Could you check a few things on this model? Use its own coordinates, in mm. A direction names the side the tool comes from. Round coordinates to 2 decimals unless told otherwise and drop trailing zeros. Order: outer loops, then holes, each group sorted by start corner. A loop starts at its lowest first (then second) coordinate and runs counter-clockwise, first axis right, second up. Notation, with made-up numbers: (39, -22.75) - (54, -22.75) arc R17 cw to (54, 3.25) - close; hole circle Ø8 at (45.5, 15). An arc over 180 degrees is marked (long way). Return JSON: item names as keys, results as strings. Group by question number.
Autodesk Fusion 360 part; units mm, degrees
sketch "Sketch1" plane through (0, 0, 0) normal (0, 1, 0) x (1, 0, 0)
  line L0 (0, 0) -> (-17.5, 0)
  line L1 (-17.5, 0) -> (-17.5, -17.5)
  line L2 (-17.5, -17.5) -> (0, -17.5)
  line L3 (0, -17.5) -> (0, 0)
  dimension "d1" = 17.5
  dimension "d2" = 17.5
extrude "Extrude1" add sketch "Sketch1" along normal blind 11
sketch "Sketch2" plane through (0, 11, 0) normal (0, 1, 0) x (-1, 0, 0)
  line L0 (0, 17.5) -> (0, 0)
  line L1 (0, 0) -> (17.5, 0)
  line L2 (17.5, 0) -> (17.5, 17.5)
  line L3 (17.5, 17.5) -> (0, 17.5)
  line L4 (7.85, 9.3) -> (9.65, 9.3)
  line L5 (9.65, 9.3) -> (9.65, 8.2)
  line L6 (9.65, 8.2) -> (7.85, 8.2)
  line L7 (7.85, 8.2) -> (7.85, 9.3)
  line L8 (8.75, 9.3) -> (8.75, 8.2)
  line L9 (9.65, 8.75) -> (7.85, 8.75)
  line L10 (0, 17.5) -> (17.5, 17.5)
  line L11 (0, 17.5) -> (0, 0)
  line L12 (8.75, 17.5) -> (8.75, 0)
  line L13 (0, 8.75) -> (17.5, 8.75)
  dimension "d5" = 1.8
  dimension "d6" = 1.1
extrude "Extrude2" add sketch "Sketch2" along normal blind 8 contours L6 L7 L8 L9 L12 L13 | L4 L7 L8 L9 L12 L13 | L4 L5 L8 L9 L12 L13 | L5 L6 L8 L9 L12 L13
sketch "Sketch3" plane through (0, 0, 0) normal (1, 0, 0) x (0, 1, 0)
  line L0 (0, 17.5) -> (0, 0)
  line L1 (0, 0) -> (11, 0)
  line L2 (11, 0) -> (11, 17.5)
  line L3 (11, 17.5) -> (0, 17.5)
  line L4 (0, 13.75) -> (11, 13.75)
  line L5 (11, 13.75) -> (11, 3.75)
  line L6 (11, 3.75) -> (0, 3.75)
  line L7 (0, 3.75) -> (0, 13.75)
  line L8 (11, 8.75) -> (0, 8.75)
  line L9 (11, 17.5) -> (11, 0)
  line L10 (11, 8.75) -> (0, 8.75)
  dimension "d11" = 10
  dimension "d12" = 11
extrude "Extrude3" add sketch "Sketch3" along normal blind 3.5 contours L0 L2 L4 L5 L7 L8 L9 L10 | L0 L2 L5 L6 L7 L8 L9 L10
sketch "Sketch4" plane through (0, 0, 17.5) normal (0, 0, 1) x (-1, 0, 0)
  line L0 (17.5, 0) -> (0, 0)
  line L1 (0, 0) -> (0, -11)
  line L2 (0, -11) -> (17.5, -11)
  line L3 (17.5, -11) -> (17.5, 0)
  line L4 (14.25, -11) -> (3.25, -11)
  line L5 (3.25, -11) -> (3.25, 0)
  line L6 (3.25, 0) -> (14.25, 0)
  line L7 (14.25, 0) -> (14.25, -11)
  line L8 (8.75, -11) -> (8.75, 0)
  line L9 (17.5, -11) -> (0, -11)
  line L10 (8.75, -11) -> (8.75, 0)
  dimension "d18" = 11
extrude "Extrude4" add sketch "Sketch4" along normal blind 3.5 contours L0 L2 L4 L6 L7 L8 L9 L10 | L0 L2 L4 L5 L6 L8 L9 L10
sketch "Sketch5" plane through (0, 0, 0) normal (0, -1, 0) x (1, 0, 0)
  line L0 (0, 13.75) -> (0, 17.5)
  line L1 (0, 17.5) -> (-3.25, 17.5)
  line L2 (-3.25, 17.5) -> (-3.25, 21)
  line L3 (-3.25, 21) -> (-14.25, 21)
  line L4 (-14.25, 21) -> (-14.25, 17.5)
  line L5 (-14.25, 17.5) -> (-17.5, 17.5)
  line L6 (-17.5, 17.5) -> (-17.5, 0)
  line L7 (-17.5, 0) -> (0, 0)
  line L8 (0, 0) -> (0, 3.75)
  line L9 (0, 3.75) -> (3.5, 3.75)
  line L10 (3.5, 3.75) -> (3.5, 13.75)
  line L11 (3.5, 13.75) -> (0, 13.75)
  line L12 (-13.45, 20.7) -> (-4.05, 20.7)
  line L13 (-4.05, 20.7) -> (-4.05, 17.8)
  line L14 (-4.05, 17.8) -> (-13.45, 17.8)
  line L15 (-13.45, 17.8) -> (-13.45, 20.7)
  line L16 (0.3, 12.95) -> (3.2, 12.95)
  line L17 (3.2, 12.95) -> (3.2, 4.55)
  line L18 (3.2, 4.55) -> (0.3, 4.55)
  line L19 (0.3, 4.55) -> (0.3, 12.95)
  line L20 (0, 17.5) -> (0, 0)
  line L21 (-17.5, 17.5) -> (0, 17.5)
  dimension "d21" = 0.8
  dimension "d22" = 0.8
  dimension "d23" = 0.8
  dimension "d24" = 0.8
  dimension "d25" = 0.3
  dimension "d27" = 0.3
  dimension "d28" = 0.3
  dimension "d29" = 0.3
extrude "Extrude5" add sketch "Sketch5" along normal blind 3.5 contours L12 L13 L14 L15 | L16 L17 L18 L19
equation "d21 = d23"
equation "d22 = d23"
equation "d24 = d23"
equation "d27 = d25"
equation "d28 = d25"
equation "d29 = d25"
1) I want a section at C-C, the plane y = 4.25. List the corners of the cut face in (x, z) for me.
2) For faces 1 (the flat face through (2, -2, 4.55)), 2 (the flat face through (-9, 15, 9.3)), 3 (the flat face through (-7.85, 15, 9)), which set-ups out of +Z, -Z, +X, -X, +Y, -Y let a thin tool reach every point of the face, with its end or its side?
3) I want a section at A-A, the plane x = 1.25. List the corners of the cut face in (y, z) for me.
4) Will these pins go through, and if not, where does the flat tip stop? pin 1 (1 mm diameter, centred on x = -5, z = 7.5, fed in from -Y); pin 2 (0.9 mm diameter, centred on y = -2, z = 19.5, fed in from +X); pin 3 (4 mm diameter, centred on x = -2, z = 8.5, fed in from +Y); pin 4 (12 mm diameter, centred on y = 14, z = 13.5, fed in from +X).
5) I want a section at B-B, the plane z = 8.5. List the corners of the cut face in (x, y) for me, plus the area to 3 significant figures.
6) If I drill on line 1 along X through (y, z) = (13, 9); line 2 along Y through (x, z) = (-8.5, 16.25); line 3 along Y through (x, z) = (-5.75, 19.75), over which ranges is the centre line in solid material (lowest first)? Write a range as from..to.
7) I want a section at D-D, the plane x = -12. List the corners of the cut face in (y, z) for me, plus the area to 3 significant figures.
Outcome:
{
 "1": {"outline": "(-17.5, 0) - (0, 0) - (0, 3.75) - (3.5, 3.75) - (3.5, 13.75) - (0, 13.75) - (0, 17.5) - (-3.25, 17.5) - (-3.25, 21) - (-14.25, 21) - (-14.25, 17.5) - (-17.5, 17.5) - close"},
 "2": {"face 1": "-Z, +X, -X, -Y", "face 2": "+Z, +X, -X, +Y", "face 3": "+Z, -Z, +X, +Y"},
 "3": {"outline": "(-3.5, 4.55) - (0, 4.55) - (0, 3.75) - (11, 3.75) - (11, 13.75) - (0, 13.75) - (0, 12.95) - (-3.5, 12.95) - close"},
 "4": {"pin 1": "y = 0", "pin 2": "x = -4.05", "pin 3": "y = 11", "pin 4": "x = 3.5"},
 "5": {"outline": "(-17.5, 0) - (0.3, 0) - (0.3, -3.5) - (3.2, -3.5) - (3.2, 0) - (3.5, 0) - (3.5, 11) - (-7.85, 11) - (-7.85, 19) - (-9.65, 19) - (-9.65, 11) - (-17.5, 11) - close", "area": "256 mm^2"},
 "6": {"line 1": "-9.65..-7.85", "line 2": "0..11", "line 3": "-3.5..11"},
 "7": {"outline": "(-3.5, 17.8) - (0, 17.8) - (0, 0) - (11, 0) - (11, 21) - (0, 21) - (0, 20.7) - (-3.5, 20.7) - close", "area": "241 mm^2"}
}
